Build history of the part. All positions in model axes, mm. Round coordinates to 2 decimals unless told otherwise and drop trailing zeros. Loops run counter-clockwise (first coordinate to the right, second up) from the corner with the lowest first, then second, coordinate; pieces in that order, holes last. Notation, with made-up numbers: M -6.75,38 L 25.25,38 A19 cw 25.25,60 Z; hole C 79,-6 d11. An arc over 180 degrees is marked long. Use one line per item in the form item = value. Start each with the question number.
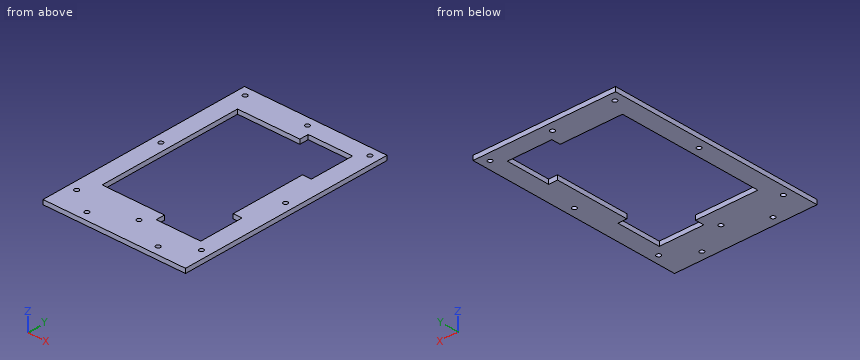
```python
from build123d import *

# Parameters (mm, degrees)
F0_R     = 3.175
F0_W     = 12.7
F0_H     = 106.4768
F0_W_2   = 203.2
F0_H_2   = 25.4
F1_DEPTH = 6.35


with BuildPart() as f1:
    # F0 (on Top) → F1 (new body)
    with BuildSketch(Plane.XY):
        Polygon((76.2, 116.7384), (101.6, 116.7384), (101.6, 142.1384), (-101.6, 142.1384), (-101.6, 116.7384), (12.7, 116.7384), (50.8, 116.7384), align=None)
        with Locations((-88.9, 129.4384)):
            Circle(F0_R, mode=Mode.SUBTRACT)
        with Locations((0, 129.4384)):
            Circle(F0_R, mode=Mode.SUBTRACT)
        with Locations((88.9, 129.4384)):
            Circle(F0_R, mode=Mode.SUBTRACT)
        Polygon((101.6, -116.7384), (76.2, -116.7384), (50.8, -116.7384), (12.7, -116.7384), (-101.6, -116.7384), (-101.6, -142.1384), (101.6, -142.1384), align=None)
        with Locations((-88.9, -129.4384)):
            Circle(F0_R, mode=Mode.SUBTRACT)
        with Locations((0, -129.4384)):
            Circle(F0_R, mode=Mode.SUBTRACT)
        with Locations((88.9, -129.4384)):
            Circle(F0_R, mode=Mode.SUBTRACT)
        Polygon((-76.2, -104.0384), (-76.2, -91.3384), (-76.2, 91.3384), (-76.2, 104.0384), (12.7, 104.0384), (12.7, 116.7384), (-101.6, 116.7384), (-101.6, -116.7384), (12.7, -116.7384), (12.7, -104.0384), align=None)
        with Locations((-88.9, 0)):
            Circle(F0_R, mode=Mode.SUBTRACT)
        Polygon((76.2, -53.2384), (76.2, -91.3384), (76.2, -104.0384), (88.9, -104.0384), (88.9, -53.2384), align=None)
        with Locations((69.85, 0)):
            Rectangle(F0_W, F0_H)
        Polygon((76.2, 91.3384), (76.2, 53.2384), (88.9, 53.2384), (88.9, 104.0384), (76.2, 104.0384), align=None)
        Polygon((76.2, 53.2384), (76.2, -53.2384), (88.9, -53.2384), (88.9, -104.0384), (76.2, -104.0384), (76.2, -116.7384), (101.6, -116.7384), (101.6, 116.7384), (76.2, 116.7384), (76.2, 104.0384), (88.9, 104.0384), (88.9, 53.2384), align=None)
        with Locations((88.9, 0)):
            Circle(F0_R, mode=Mode.SUBTRACT)
        with Locations((0, -154.8384)):
            Rectangle(F0_W_2, F0_H_2)
        with Locations((-50.8, -154.8384)):
            Circle(F0_R, mode=Mode.SUBTRACT)
        with Locations((50.8, -154.8384)):
            Circle(F0_R, mode=Mode.SUBTRACT)
    extrude(amount=F1_DEPTH)


solid = f1.part
```
Q1. Saw through at C-C (x = 31.5). Give the cut face in (y, z), and give its area (3 significant figures).
Q2. Drop flat-ended pins along their axis: P1, Ø8.5, axis at x = 88.9, y = -129.44, coming from the -Z side; P2, Ø5, axis at x = -50.8, y = -154.84, coming from the -Z side. Give the stop position or say it passes through.
Q3. Wall check: probe 1 along X at (y, z) = (-155, 3.25); probe 2 along Y at (x, z) = (65, 2.25); probe 3 along X at (y, z) = (-18, 1). Give the ranges that are in metal, low to high.
Q4. Saw through at B-B (x = 0). Give the cut face in (y, z), and give its area (3 significant figures).
Q5. Saw through at A-A (y = 0). Give the cut face in (x, z) (3 decimals), and give its area (3 significant figures).
Q6. Saw through at D-D (z = 4.25). Give the number of separate pieces and of enclosed holes in the cut face, and give its area (3 significant figures).
Filled in:
q1.outline = M -167.54,0 L -116.74,0 L -116.74,6.35 L -167.54,6.35 Z; M 116.74,0 L 142.14,0 L 142.14,6.35 L 116.74,6.35 Z
q1.area = 484 mm²
q2.P1 = 0
q2.P2 = through
q3.probe_1 = -101.6 to -53.97, -47.63 to 47.63, 53.97 to 101.6
q3.probe_2 = -167.54 to -116.74, -53.24 to 53.24, 116.74 to 142.14
q3.probe_3 = -101.6 to -76.2, 63.5 to 101.6
q4.outline = M -167.54,0 L -132.61,0 L -132.61,6.35 L -167.54,6.35 Z; M -126.26,0 L -104.04,0 L -104.04,6.35 L -126.26,6.35 Z; M 104.04,0 L 126.26,0 L 126.26,6.35 L 104.04,6.35 Z; M 132.61,0 L 142.14,0 L 142.14,6.35 L 132.61,6.35 Z
q4.area = 565 mm²
q5.outline = M -101.6,0 L -92.075,0 L -92.075,6.35 L -101.6,6.35 Z; M -85.725,0 L -76.2,0 L -76.2,6.35 L -85.725,6.35 Z; M 63.5,0 L 85.725,0 L 85.725,6.35 L 63.5,6.35 Z; M 92.075,0 L 101.6,0 L 101.6,6.35 L 92.075,6.35 Z
q5.area = 323 mm²
q6.separate_pieces = 1
q6.enclosed_holes = 11
q6.area = 30,600 mm²
